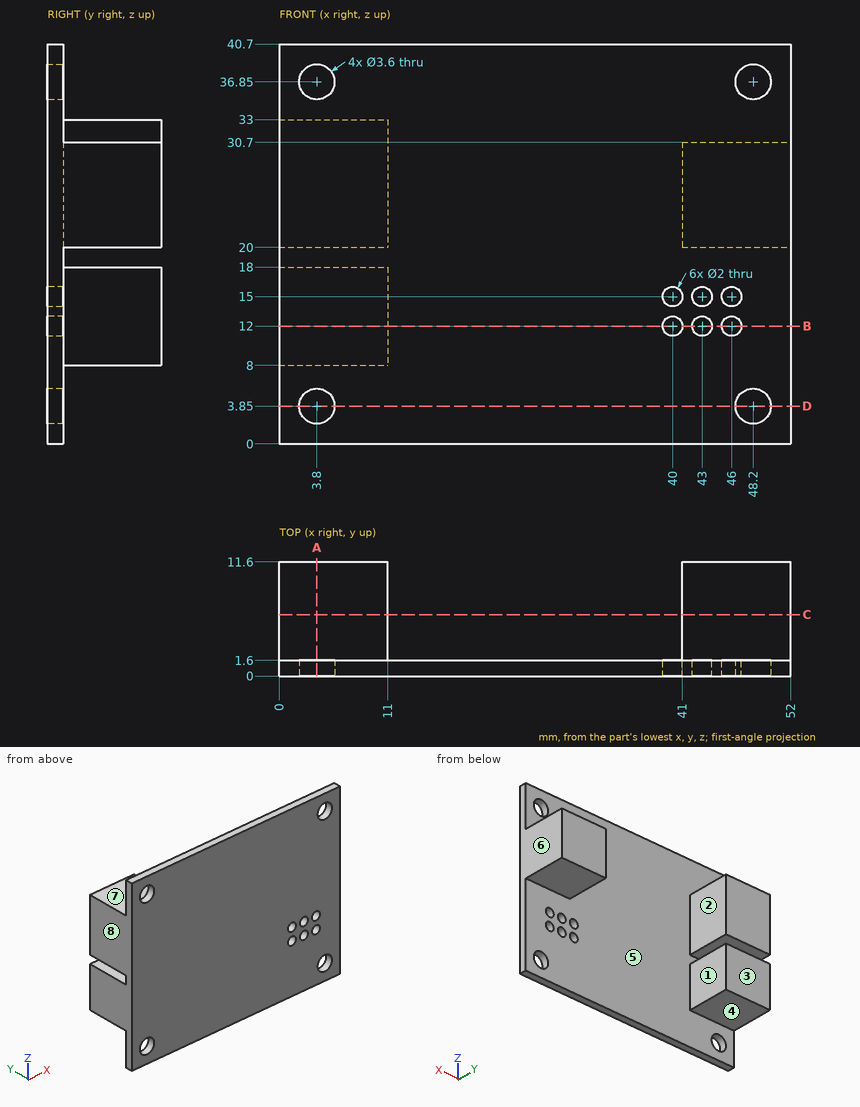
The drawing under review shows one solid part. Ordinate dimensions are in mm from its lowest x, y, z. A direction names the side the tool comes from. Give positions to 0.01 mm unless a question says otherwise; leave off trailing zeros. Write each loop counter-clockwise with the first axis right and the second up, starting at its lowest first coordinate (ties: lowest second). Pieces come first, ordered by that corner, then holes. Notation, with made-up numbers: (-16, -6) - (-5, -6) arc R21 ccw to (-5, 4) - close; hole circle Ø6 at (82.25, -21.5). An arc over 180 degrees is marked (long way). Answer in a Markdown table with one row per item. Add a question column.
1. We need section B-B on z = 12. Write out the cut boundary in (x, y), then the cut area to 3 significant figures.
2. Wall thickness on line 1 along X through (y, z) = (1.05, 12); line 2 along Z through (x, y) = (40, 1.5); line 3 along X through (y, z) = (1.25, 4): over which ranges is each line inside the solid? List them lowest first. Write a range as [from, to].
3. Draft analysis for pull direction X (two halves, no side actions). For the marked faces 5, 6, 7 and 8, state which applies: +X half, -X half, draft (parallel to the pull), parting line (faces both ways), or undercut.
4. We need section D-D on z = 3.85. Write out the cut boundary in (x, y), then the cut area to 3 significant figures.
5. We need section A-A on x = 3.8. Write out the cut boundary in (y, z).
6. Tool access review of the marked faces 1, 2, 3 and 4: name each direction out of +Z, -Z, +X, -X, +Y, -Y from which nothing blocks a thin tool from reaching the whole face with its end or side.
7. We need section C-C on y = 6.25. Write out the cut boundary in (x, z).
8. Insertion check: P1, Ø20.5, axis at x = 27.5, z = 13, coming from the +Y side; P2, Ø2, axis at x = 41, y = 10.5, coming from the -Z side; P3, Ø3, axis at x = 6, y = 4.5, coming from the +Z side. Each pin has a flat end and moves straight along its axis. Give the tip position at first contact, or say it passes through.
Ans:
| question | item | result |
|---|---|---|
| 1 | outline | (0, 0) - (39, 0) - (39, 1.6) - (11, 1.6) - (11, 11.6) - (0, 11.6) - close; (41, 0) - (42, 0) - (42, 1.6) - (41, 1.6) - close; (44, 0) - (45, 0) - (45, 1.6) - (44, 1.6) - close; (47, 0) - (52, 0) - (52, 1.6) - (47, 1.6) - close |
| 1 | area | 184 mm^2 |
| 2 | line 1 | x = [0, 39], [41, 42], [44, 45], [47, 52] |
| 2 | line 2 | z = [0, 11], [13, 14], [16, 40.7] |
| 2 | line 3 | x = [0, 2.01], [5.59, 46.41], [49.99, 52] |
| 3 | face 5 | undercut |
| 3 | face 6 | +X half |
| 3 | face 7 | draft |
| 3 | face 8 | -X half |
| 4 | outline | (0, 0) - (2, 0) - (2, 1.6) - (0, 1.6) - close; (5.6, 0) - (46.4, 0) - (46.4, 1.6) - (5.6, 1.6) - close; (50, 0) - (52, 0) - (52, 1.6) - (50, 1.6) - close |
| 4 | area | 71.7 mm^2 |
| 5 | outline | (0, 0) - (1.6, 0) - (1.6, 2.05) - (0, 2.05) - close; (0, 5.65) - (1.6, 5.65) - (1.6, 8) - (11.6, 8) - (11.6, 18) - (1.6, 18) - (1.6, 20) - (11.6, 20) - (11.6, 33) - (1.6, 33) - (1.6, 35.05) - (0, 35.05) - close; (0, 38.65) - (1.6, 38.65) - (1.6, 40.7) - (0, 40.7) - close |
| 6 | face 1 | +Z, -Z, +X, +Y |
| 6 | face 2 | +Z, -Z, +Y |
| 6 | face 3 | +Z, -Z, +X, -X, +Y |
| 6 | face 4 | -Z, +X, -X, +Y |
| 7 | outline | (0, 8) - (11, 8) - (11, 18) - (0, 18) - close; (0, 20) - (11, 20) - (11, 33) - (0, 33) - close; (41, 20) - (52, 20) - (52, 30.7) - (41, 30.7) - close |
| 8 | P1 | stops at y = 1.6 |
| 8 | P2 | stops at z = 20 |
| 8 | P3 | stops at z = 33 |
